Can you work these out from the model? Positions are in its coordinate system, mm. A direction names the side the tool comes from. Give positions to 0.01 mm unless a question says otherwise; leave off trailing zeros. Loops run counter-clockwise (first coordinate to the right, second up) from the corner with the lowest first, then second, coordinate; pieces in that order, holes last. Notation, with made-up numbers: (-2.5, 5.5) - (19.5, 5.5) arc R22 ccw to (19.5, 44.5) - close; hole circle Ø6 at (-8.75, -27). An arc over 180 degrees is marked (long way). Use a Markdown table: item, result. Add a question column.
Solid Edge part; units mm, degrees
sketch "Sketch1" plane through (0, 0, 0) normal (0, 0, -1) x (-1, 0, 0)
  line L0 (-85.725, -85.725) -> (85.725, -85.725)
  line L1 (85.725, -85.725) -> (85.725, 85.725)
  line L2 (85.725, 85.725) -> (-85.725, 85.725)
  line L3 (-85.725, 85.725) -> (-85.725, -85.725)
extrude "ExtrudedProtrusion_18" add sketch "Sketch1" along normal blind 4
sketch "Sketch2" plane through (0, 0, -4) normal (0, 0, -1) x (0, -1, 0)
  line L0 (-70.0986, 45) -> (-70.0986, -45)
  arc A0 (-70.0986, -45) -> (-40.0986, -75) centre (-40.0986, -45) ccw
  line L1 (18.055, -75) -> (-40.0986, -75)
  arc A1 (18.055, -75) -> (48.055, -45) centre (18.055, -45) ccw
  line L2 (48.055, -45) -> (48.055, 45)
  arc A2 (18.055, 75) -> (48.055, 45) centre (18.055, 45) cw
  line L3 (-40.0986, 75) -> (18.055, 75)
  arc A3 (-40.0986, 75) -> (-70.0986, 45) centre (-40.0986, 45) ccw
  dimension "D1" = 70.0986
extrude "Cutout1" cut sketch "Sketch2" against normal blind 18
sketch "Sketch3" plane through (-85.725, 77.9118, -2) normal (-1, 0, 0) x (0, -1, 0)
  line L0 (-7.8132, 2) -> (163.6368, 2)
  line L1 (163.6368, 2) -> (163.6368, -2)
  line L2 (163.6368, -2) -> (-7.8132, -2)
  line L3 (-7.8132, -2) -> (-7.8132, 2)
extrude "ExtrudedProtrusion_19" add sketch "Sketch3" along normal blind 15
sketch "Sketch4" plane through (85.725, -66.89, -2) normal (1, 0, 0) x (0, -1, 0)
  line L0 (-152.615, 2) -> (18.835, 2)
  line L1 (18.835, 2) -> (18.835, -2)
  line L2 (18.835, -2) -> (-152.615, -2)
  line L3 (-152.615, -2) -> (-152.615, 2)
extrude "Protrusion1" add sketch "Sketch4" along normal blind 15
sketch "Sketch5" plane through (0, 0, -4) normal (0, 0, -1) x (0, 1, 0)
  line L0 (85.725, 100.725) -> (65.725, 100.725)
  line L1 (65.725, 100.725) -> (65.725, 87.725)
  line L2 (65.725, 87.725) -> (85.725, 87.725)
  line L3 (85.725, 87.725) -> (85.725, 100.725)
  line L4 (85.725, -100.725) -> (65.725, -100.725)
  line L5 (65.725, -100.725) -> (65.725, -87.725)
  line L6 (65.725, -87.725) -> (85.725, -87.725)
  line L7 (85.725, -87.725) -> (85.725, -100.725)
extrude "Cutout2" cut sketch "Sketch5" against normal blind 20
sketch "Sketch6" plane through (0, 0.5, -4) normal (0, 0, -1) x (0, -1, 0)
  circle A0 centre (79.8229, 79.4583) radius 2
  circle A1 centre (-78.6752, -79.8014) radius 2
  circle A2 centre (53.349, -79.9109) radius 2
  circle A3 centre (-78.6746, 79.5467) radius 2.0294
extrude "ExtrudedCutout_38" cut sketch "Sketch6" against normal blind 50
sketch "Sketch7" plane through (100.725, -10, 6) normal (1, 0, 0) x (0, -1, 0)
  line L0 (75.725, 10) -> (55.725, 10)
  line L1 (55.725, 10) -> (55.725, 6)
  line L2 (55.725, 6) -> (75.725, 6)
  line L3 (75.725, 6) -> (75.725, 10)
extrude "ExtrudedProtrusion_23" add sketch "Sketch7" along normal mid plane 6
sketch "Sketch8" plane through (-100.725, -10, 6) normal (-1, 0, 0) x (0, 1, 0)
  line L0 (-75.725, 10) -> (-55.725, 10)
  line L1 (-55.725, 10) -> (-55.725, 6)
  line L2 (-55.725, 6) -> (-75.725, 6)
  line L3 (-75.725, 6) -> (-75.725, 10)
extrude "ExtrudedProtrusion_24" add sketch "Sketch8" along normal mid plane 6
sketch "Sketch9" plane through (-94.225, 65.725, -2) normal (0, 1, 0) x (0, 0, -1)
  line L0 (-2, -197.95) -> (-1, -197.95)
  line L1 (-1, -197.95) -> (-1, 28.925)
  line L2 (-1, 28.925) -> (-2, 28.925)
  line L3 (-2, 28.925) -> (-2, -197.95)
extrude "Cutout3" cut sketch "Sketch9" against normal blind 555
sketch "Sketch10" plane through (0, 0, -4) normal (0, 0, -1) x (1, 0, 0)
  line L0 (87.725, -65.725) -> (97.725, -65.725)
  line L1 (97.725, -65.725) -> (97.725, -85.725)
  line L2 (97.725, -85.725) -> (87.725, -85.725)
  line L3 (87.725, -85.725) -> (87.725, -65.725)
  line L4 (-87.725, -65.725) -> (-97.725, -65.725)
  line L5 (-97.725, -65.725) -> (-97.725, -85.725)
  line L6 (-97.725, -85.725) -> (-87.725, -85.725)
  line L7 (-87.725, -85.725) -> (-87.725, -65.725)
extrude "Protrusion2" add sketch "Sketch10" against normal blind 3
1. If we mould it in two halves opening along X, with no side actions, what happens to faces 1 (the face through (-66.445, 61.077, -2.472)), 2 (the face through (-80.16, 77.24, -2.03)), 3 (the face through (1, 78, 0))? For each: released by +X, released by -X, zero draft, split by the parting line, or undercut.
2. Suppose I cut it at C-C (z = -2.1). List the corners of the cut face in (x, y) for me (3 decimals), and give its area (3 significant figures).
3. Suppose I cut it at A-A (y = 25). List the corners of the cut face in (x, z) for me (3 decimals).
4. Will these pins go through, and if not, where does the flat tip stop? P1, Ø1.5, axis at y = 50, z = -2.5, coming from the +X side (3 decimals); P2, Ø6.5, axis at x = -79.46, y = -79.32, coming from the +Z side; P3, Ø2, axis at x = -18.5, y = -47, coming from the -Z side; P4, Ø0.5, axis at y = 76.5, z = -0.5, coming from the +X side (3 decimals).
5. On a 3-axis mill with a long thin cutter (end or side, diameter ignored), from which of +Z, -Z, +X, -X, +Y, -Y can I reach the whole of each face in a straight line? I mean faces 4 (the face through (66.45, -39.03, -2.52)), 5 (the face through (1, -56, -4)). Say none if no direction works.
6. Suppose I cut it at B-B (x = -2.5). List the corners of the cut face in (y, z) for me (3 decimals).
7. Please list where these lines run through material, in increasing order: line 1 along Y through (x, z) = (11, -3.7) (3 decimals); line 2 along X through (y, z) = (-3, -3.2) (3 decimals); line 3 along X through (y, z) = (-29, -2.35) (3 decimals). Write a range as [from, to].
8. Suppose I cut it at D-D (y = -73). List the corners of the cut face in (x, z) for me (3 decimals), and give its area (3 significant figures).
Results below:
| question | item | result |
|---|---|---|
| 1 | face 1 | undercut |
| 1 | face 2 | undercut |
| 1 | face 3 | zero draft |
| 2 | outline | (-103.725, -85.725) - (103.725, -85.725) - (103.725, -65.725) - (100.725, -65.725) - (100.725, 65.725) - (97.725, 65.725) - (97.725, 85.725) - (-97.725, 85.725) - (-97.725, 65.725) - (-100.725, 65.725) - (-100.725, -65.725) - (-103.725, -65.725) - close; hole circle Ø4.059 at (-79.547, 79.175); hole circle Ø4 at (-79.458, -79.323); hole (-75, -18.055) arc R30 ccw to (-45, -48.055) - (45, -48.055) arc R30 ccw to (75, -18.055) - (75, 40.099) arc R30 ccw to (45, 70.099) - (-45, 70.099) arc R30 ccw to (-75, 40.099) - close; hole circle Ø4 at (79.801, 79.175); hole circle Ø4 at (79.911, -52.849) |
| 2 | area | 17,500 mm² |
| 3 | outline | (-100.725, -4) - (-75, -4) - (-75, -1) - (-100.725, -1) - close; (75, -4) - (100.725, -4) - (100.725, -1) - (75, -1) - close |
| 4 | P1 | x = 100.725 |
| 4 | P2 | z = -1 |
| 4 | P3 | through |
| 4 | P4 | x = 87.725 |
| 5 | face 4 | +Z, -Z |
| 5 | face 5 | -Z, +X, -X, +Y, -Y |
| 6 | outline | (-85.725, -4) - (-48.055, -4) - (-48.055, -1) - (-85.725, -1) - close; (70.099, -4) - (85.725, -4) - (85.725, 0) - (70.099, 0) - close |
| 7 | line 1 | [-85.725, -48.055], [70.099, 85.725] |
| 7 | line 2 | [-100.725, -75], [75, 100.725] |
| 7 | line 3 | [-100.725, -72.932], [72.932, 100.725] |
| 8 | outline | (-103.725, -4) - (103.725, -4) - (103.725, -1) - (-103.725, -1) - close |
| 8 | area | 622 mm² |
